Can you work these out from the model? Positions are in its coordinate system, mm. Face numbers are marked on the shaded views. Give positions to 0.01 mm unless a question says otherwise; leave off trailing zeros. Write each loop counter-clockwise with the first axis right and the second up, starting at its lowest first coordinate (ties: lowest second). Pieces come first, ordered by that corner, then holes.
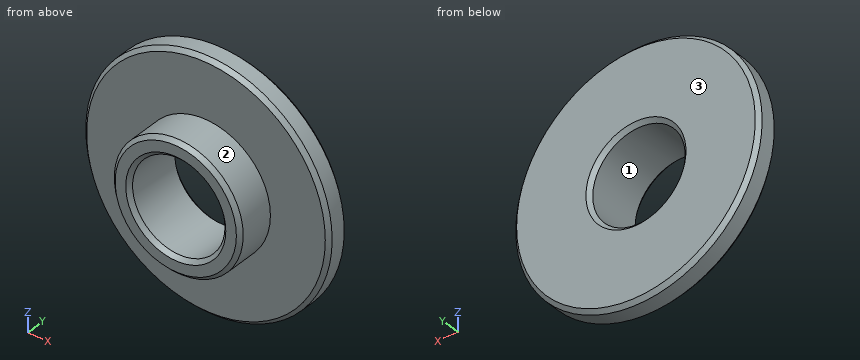
```python
from build123d import *

# Parameters (mm, degrees)
F0_R     = 16
F0_R_2   = 8.375
F0_R_3   = 6
F1_DEPTH = 3
F2_DEPTH = 8
F3_SIZE  = 0.5


with BuildPart() as f1:
    # F0 (on Front) → F1 (new body)
    with BuildSketch(Plane.XZ):
        Circle(F0_R)
        Circle(F0_R_2, mode=Mode.SUBTRACT)
        Circle(F0_R_2)
        Circle(F0_R_3, mode=Mode.SUBTRACT)
    extrude(amount=F1_DEPTH)

    # F0 (on Front) → F2 (join)
    with BuildSketch(Plane.XZ):
        Circle(F0_R_2)
        Circle(F0_R_3, mode=Mode.SUBTRACT)
    extrude(amount=F2_DEPTH)

    # F3
    f3_edges = [f1.edges().sort_by_distance(p)[0] for p in [
        (16, -1.5, 0),
        (-16, 0, 0),
        (-16, -3, 0),
        (-6, 0, 0),
        (6, -4, 0),
        (-6, -8, 0),
        (-8.375, -8, 0),
    ]]
    chamfer(f3_edges, length=F3_SIZE)


solid = f1.part
```
1) Suppose I cut it at A-A on x = 0. Write out the boundary of the cut face in (y, z) (3 decimals), plus the area to 3 significant figures.
Values follow:
outline: (-8, -7.875) - (-7.5, -8.375) - (-3, -8.375) - (-3, -15.5) - (-2.5, -16) - (-0.5, -16) - (0, -15.5) - (0, -6.5) - (-0.5, -6) - (-7.5, -6) - (-8, -6.5) - close; (-8, 6.5) - (-7.5, 6) - (-0.5, 6) - (0, 6.5) - (0, 15.5) - (-0.5, 16) - (-2.5, 16) - (-3, 15.5) - (-3, 8.375) - (-7.5, 8.375) - (-8, 7.875) - close
area: 82.5 mm2
2) If we mould it in two halves opening along Z, with no side actions, what happens to the marked faces 1, 2 and 3? For each: +Z half, -Z half, draft (parallel to the pull), parting line (faces both ways), or undercut.
Values follow:
face 1: undercut
face 2: parting line
face 3: draft
3) Suppose I cut it at C-C on y = -4.5. Write out the boundary of the cut face in (x, z) (3 decimals).
Values follow:
outline: circle Ø16.75 at (0, 0); hole circle Ø12 at (0, 0)
4) Suppose I cut it at D-D on y = -1. Write out the boundary of the cut face in (x, z), plus the area to 3 significant figures.
Values follow:
outline: circle Ø32 at (0, 0); hole circle Ø12 at (0, 0)
area: 691 mm2
5) Please list where these lines run through material, in increasing order: L1, parallel to Z at x = 0, y = -5.5 (3 decimals); L2, parallel to Y at x = -10, z = 10; L3, parallel to Z at x = 0, y = -2.
Values follow:
L1: z = -8.375 to -6, 6 to 8.375
L2: y = -3 to 0
L3: z = -16 to -6, 6 to 16
6) For pin 1 Ø1 at (x, z) = (2.5, 9) entering from -Y; pin 2 Ø4 at (x, y) = (1, -6) entering from -Z (3 decimals); pin 3 Ø2 at (y, z) = (-1, -12.5) entering from -X; pin 4 Ø9.5 at (x, z) = (0, 0) entering from +Y, each with a flat end and sliding along its axis, tell me the tip position at first contact or that it passes through.
Values follow:
pin 1: stops at y = -3
pin 2: stops at z = -8.375
pin 3: stops at x = -11.12
pin 4: passes through
7) Suppose I cut it at B-B on z = 0. Write out the boundary of the cut face in (x, y) (3 decimals).
Values follow:
outline: (-16, -2.5) - (-15.5, -3) - (-8.375, -3) - (-8.375, -7.5) - (-7.875, -8) - (-6.5, -8) - (-6, -7.5) - (-6, -0.5) - (-6.5, 0) - (-15.5, 0) - (-16, -0.5) - close; (6, -7.5) - (6.5, -8) - (7.875, -8) - (8.375, -7.5) - (8.375, -3) - (15.5, -3) - (16, -2.5) - (16, -0.5) - (15.5, 0) - (6.5, 0) - (6, -0.5) - close
